Could you check a few things on this drawing? It's one solid part, dimensions in mm from its lowest x, y, z. Give positions to 0.01 mm unless a question says otherwise; leave off trailing zeros. Write each loop counter-clockwise with the first axis right and the second up, starting at its lowest first coordinate (ties: lowest second). Pieces come first, ordered by that corner, then holes. Notation, with made-up numbers: M -40,21.25 L 17,21.25 A19 cw 17,26.25 Z; hole C -14.5,52 d6. An arc over 180 degrees is marked long. Write each question's results on one line, items separated by ' | '. Start each with the question number.
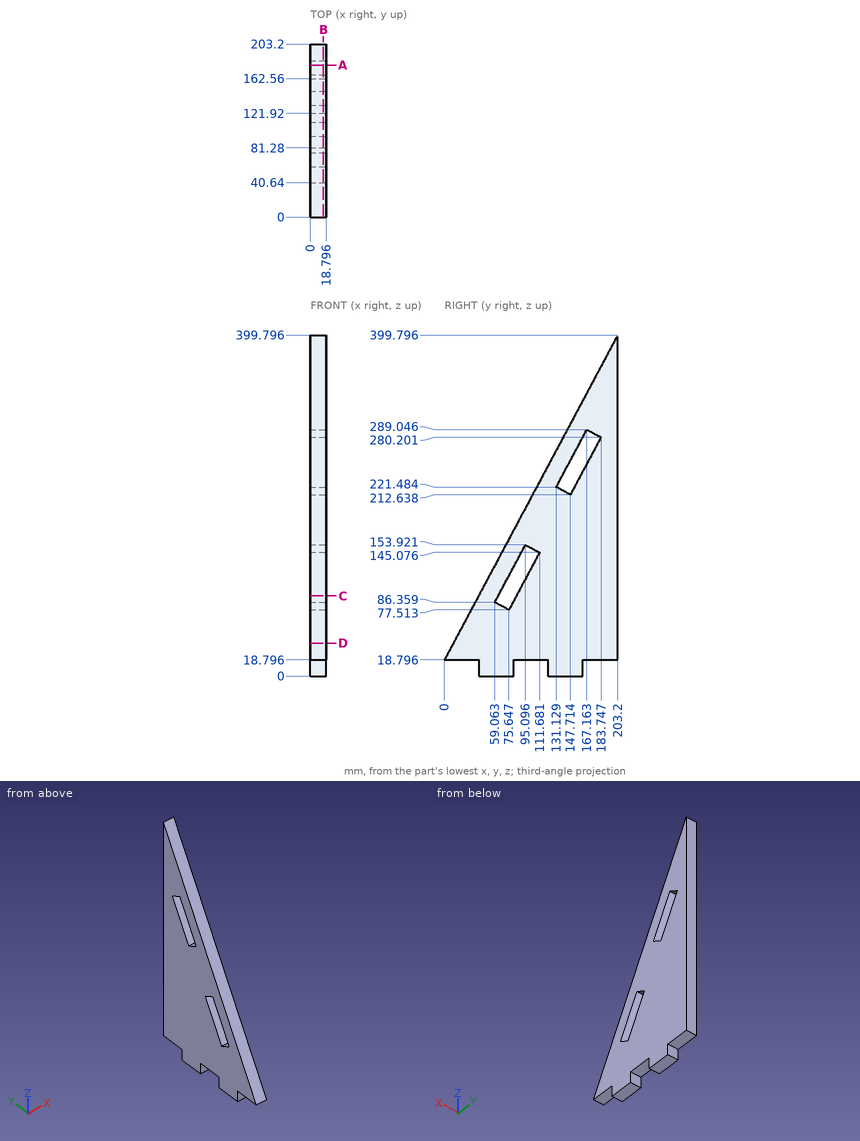
Q1. If we section it at B-B (x = 15.25): Please give me the cut outline in (y, z) (1 decimal), plus the area to 3 significant figures.
Q2. If we section it at A-A (y = 178.5): Please give me the cut outline in (x, z), plus the area to 3 significant figures.
Q3. I'm going to push flat-ended pins straight in: P1, Ø9.5, axis at x = 12, y = 191, coming from the -Z side; P2, Ø6, axis at x = 13.5, y = 178.5, coming from the +Z side; P3, Ø8, axis at x = 6.5, y = 83.5, coming from the -Z side; P4, Ø5.5, axis at x = 5, z = 11.5, coming from the +Y side. Where does each tip first touch, or does it pass through?
Q4. If we section it at D-D (z = 38.5): Please give me the cut outline in (x, y).
Q5. Please list where these lines run through material, in increasing order: line 1 (Y direction, x = 1.5, z = 277); line 2 (Z direction, x = 16.5, y = 76) (1 decimal); line 3 (Y direction, x = 16, z = 280). Write a range as [from, to].
Q6. If we section it at C-C (z = 94): Please give me the cut outline in (x, y), plus the area to 4 significant figures.
Determined:
1) outline: M 0,18.8 L 40.6,18.8 L 40.6,0 L 81.3,0 L 81.3,18.8 L 121.9,18.8 L 121.9,0 L 162.6,0 L 162.6,18.8 L 203.2,18.8 L 203.2,399.8 Z; hole M 59.1,86.4 L 75.6,77.5 L 111.7,145.1 L 95.1,153.9 Z; hole M 131.1,221.5 L 147.7,212.6 L 183.7,280.2 L 167.2,289 Z | area: 37,400 mm²
2) outline: M 0,18.8 L 18.8,18.8 L 18.8,270.36 L 0,270.36 Z; M 0,283 L 18.8,283 L 18.8,353.48 L 0,353.48 Z | area: 6,050 mm²
3) P1: stops at z = 18.8 | P2: stops at z = 359.11 | P3: stops at z = 0 | P4: stops at y = 162.56
4) outline: M 0,10.51 L 18.8,10.51 L 18.8,203.2 L 0,203.2 Z
5) line 1: y = [137.71, 160.74], [182.04, 203.2] | line 2: z = [0, 78.2], [118.1, 161.3] | line 3: y = [139.31, 162.34], [183.64, 203.2]
6) outline: M 0,40.11 L 18.8,40.11 L 18.8,63.14 L 0,63.14 Z; M 0,84.44 L 18.8,84.44 L 18.8,203.2 L 0,203.2 Z | area: 2,665 mm²
